Part model, mm, in its own coordinate system. A direction names the side the tool comes from. Give positions to 0.01 mm unless a question says otherwise; leave off trailing zeros. Order: outer loops, then holes, each group sorted by start corner. A loop starts at its lowest first (then second) coordinate and runs counter-clockwise, first axis right, second up.
1. Probe line 1 (X direction, y = 1.6, z = -11); line 2 (X direction, y = 0.6, z = -14); line 3 (X direction, y = 0.4, z = -21). List the from-to ranges inside material, lowest first.
2. Which spindle directions (+Z, -Z, +X, -X, +Y, -Y) get a long thin tool onto all of the face, cutting with end or side? Do faces 4 (the cylindrical face through (-3.773, 0.986, -12.571)), 5 (the flat face through (0, 1, -15)). Say none if no direction does.
3. Mould opens along Z. For faces 1 (the cylindrical face through (0, 1, 5)), 2 (the flat face through (1.2, 2, -6.5)), 3 (the flat face through (1, 1, -10)) say: +Z half, -Z half, draft (parallel to the pull), parting line (faces both ways), or undercut.
4. Slice it at D-D on z = -22. List the corners of the cut face in (x, y).
5. Slice it at A-A on y = 0.45. List the corners of the cut face in (x, z).
6. Slice it at C-C on x = -3.5. List the corners of the cut face in (y, z).
7. Drop flat-ended pins along their axis: pin 1 Ø1 at (x, z) = (0.5, -15) entering from -Y; pin 2 Ø1 at (y, z) = (1.5, -10.5) entering from +X; pin 3 Ø0.6 at (x, y) = (-0.5, 1) entering from -Z; pin 4 Ø1 at (y, z) = (1, -8.5) entering from -X. Give the stop position or say it passes through.
8. Slice it at B-B on z = -8. List the corners of the cut face in (x, y), and give its area (3 significant figures).
Autodesk Inventor part; units mm, degrees
ref_plane "YZ Plane" through (0, 0, 0) normal (1, 0, 0) x (0, 1, 0)
ref_plane "XZ Plane" through (0, 0, 0) normal (0, 1, 0) x (-1, 0, 0)
ref_plane "XY Plane" through (0, 0, 0) normal (0, 0, 1) x (1, 0, 0)
sketch "Sketch1" plane through (0, 0, 0) normal (0, 1, 0) x (-1, 0, 0)
  arc A0 (5, 0) -> (-5, 0) centre (0, 0) ccw
  arc A1 (0, -25) -> (5, 0) centre (-60, 0) ccw
  arc A2 (-5, 0) -> (0, -25) centre (60, 0) ccw
  circle A3 centre (0, 0) radius 1
  line L0 (1, -5) -> (-1, -5)
  line L1 (-1, -5) -> (-1, -15)
  line L2 (-1, -15) -> (1, -15)
  line L3 (1, -15) -> (1, -5)
  dimension "d0" = 5
  dimension "d1" = 0
  dimension "d2" = 0
  dimension "d3" = 0
  dimension "d4" = 0
  dimension "d5" = 0
  dimension "d6" = 25
  dimension "d7" = 2
  dimension "d10" = 10
  dimension "d11" = 2
  dimension "d12" = 1
  dimension "d13" = 5
extrude "Extrusion2" add sketch "Sketch1" along normal blind 2
properties part number "aileron_arriere"
Data:
1. line 1: x = -4.06 to -1, 1 to 4.06
1. line 2: x = -3.47 to -1, 1 to 3.47
1. line 3: x = -1.51 to 1.51
2. face 4: -Z, -X, +Y, -Y
2. face 5: +Y, -Y
3. face 1: +Z half
3. face 2: draft
3. face 3: undercut
4. outline: (-1.16, 0) - (1.16, 0) - (1.16, 2) - (-1.16, 2) - close
5. outline: (-5, 0) arc R65 ccw to (0, -25) arc R65 ccw to (5, 0) arc R5 ccw to start; hole (-1, -15) - (1, -15) - (1, -5) - (-1, -5) - close; hole circle Ø2 at (0, 0)
6. outline: (0, -13.88) - (2, -13.88) - (2, 3.57) - (0, 3.57) - close
7. pin 1: stops at y = 0
7. pin 2: stops at x = 4.23
7. pin 3: stops at z = -24.51
7. pin 4: stops at x = -4.51
8. outline: (-4.51, 0) - (-1, 0) - (-1, 2) - (-4.51, 2) - close; (1, 0) - (4.51, 0) - (4.51, 2) - (1, 2) - close
8. area: 14.0 mm2
